Verification items for the finished model (mm, model axes). Face numbers are marked on the shaded views. A direction names the side the tool comes from. Coordinates: 2 decimals unless noted, no trailing zeros. Write each loop counter-clockwise with the first axis right and the second up, starting at its lowest first coordinate (ties: lowest second). Pieces come first, ordered by that corner, then holes. Notation, with made-up numbers: (78, 15.25) -> (85, 15.25) arc R22 ccw to (85, 28.25) -> close; hole circle Ø5 at (25.25, 26). An arc over 180 degrees is marked (long way). Answer in a Markdown table with one row per item.
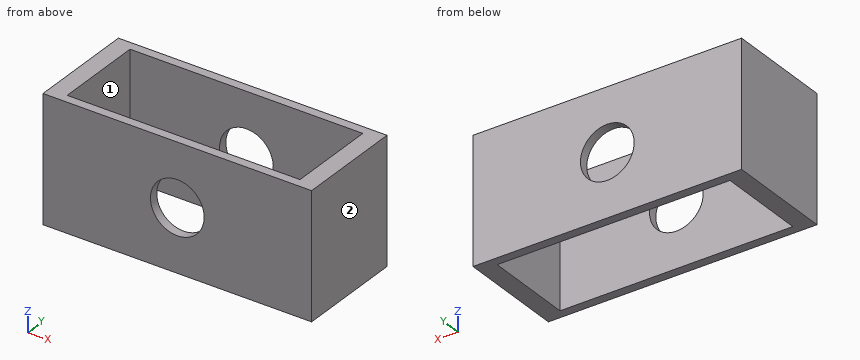
```python
from build123d import *

# Parameters (mm, degrees)
SKETCH_1_W      = 30
SKETCH_1_H      = 14
SKETCH_1_R      = 3
EXTRUDE_1_DEPTH = 1
SKETCH_2_W      = 2
SKETCH_2_H      = 14
EXTRUDE_2_DEPTH = 10
SKETCH_3_W      = 30
SKETCH_3_H      = 14
SKETCH_3_R      = 3
EXTRUDE_3_DEPTH = 1


with BuildPart() as part:
    # Эскиз1 → Бобышка-Вытянуть1 (new body)
    with BuildSketch(Plane(origin=(0, 0, 0), x_dir=(1, 0, 0), z_dir=(0, 1, 0))):
        Rectangle(SKETCH_1_W, SKETCH_1_H)
        with Locations(Location((0, 0, 0), (0, 0, 270))):
            Circle(SKETCH_1_R, mode=Mode.SUBTRACT)
    extrude(amount=EXTRUDE_1_DEPTH)

    # Эскиз2 → Бобышка-Вытянуть2 (add)
    with BuildSketch(Plane(origin=(0, 1, 0), x_dir=(1, 0, 0), z_dir=(0, 1, 0))):
        with Locations((-14, 0)):
            Rectangle(SKETCH_2_W, SKETCH_2_H)
        with Locations((14, 0)):
            Rectangle(SKETCH_2_W, SKETCH_2_H)
    extrude(amount=EXTRUDE_2_DEPTH)

    # Эскиз3 → Бобышка-Вытянуть3 (add)
    with BuildSketch(Plane(origin=(0, 11, 0), x_dir=(1, 0, 0), z_dir=(0, 1, 0))):
        Rectangle(SKETCH_3_W, SKETCH_3_H)
        with Locations(Location((0, 0, 0), (0, 0, 270))):
            Circle(SKETCH_3_R, mode=Mode.SUBTRACT)
    extrude(amount=EXTRUDE_3_DEPTH)


solid = part.part
```
1. Depth check by flat-ended pin: P1, Ø4, axis at x = 3.5, z = -4.5, coming from the -Y side; P2, Ø3.5, axis at x = 0, z = 0, coming from the -Y side. Enter the tip coordinate at first touch or a pass-through.
Geometry says:
| item | result |
|---|---|
| P1 | y = 0 |
| P2 | through |
2. Section check B-B, the plane y = 3. Record the boundary of the cut face in (x, z), plus the area to 3 significant figures.
Geometry says:
| item | result |
|---|---|
| outline | (-15, -7) -> (-13, -7) -> (-13, 7) -> (-15, 7) -> close; (13, -7) -> (15, -7) -> (15, 7) -> (13, 7) -> close |
| area | 56.0 mm^2 |
3. Section check C-C, the plane z = 0. Record the boundary of the cut face in (x, y), plus the area to 3 significant figures.
Geometry says:
| item | result |
|---|---|
| outline | (-15, 0) -> (-3, 0) -> (-3, 1) -> (-13, 1) -> (-13, 11) -> (-3, 11) -> (-3, 12) -> (-15, 12) -> close; (3, 0) -> (15, 0) -> (15, 12) -> (3, 12) -> (3, 11) -> (13, 11) -> (13, 1) -> (3, 1) -> close |
| area | 88.0 mm^2 |
4. Tool access check on the marked faces 1 and 2. Record the directions out of +Z, -Z, +X, -X, +Y, -Y that give a thin tool (end or side, any length) a straight path to the whole face; none if there is none.
Geometry says:
| item | result |
|---|---|
| face 1 | +Z, -Z |
| face 2 | +Z, -Z, +X, +Y, -Y |
5. Section check A-A, the plane x = 0. Record the boundary of the cut face in (y, z).
Geometry says:
| item | result |
|---|---|
| outline | (0, -7) -> (1, -7) -> (1, -3) -> (0, -3) -> close; (0, 3) -> (1, 3) -> (1, 7) -> (0, 7) -> close; (11, -7) -> (12, -7) -> (12, -3) -> (11, -3) -> close; (11, 3) -> (12, 3) -> (12, 7) -> (11, 7) -> close |
6. Section check D-D, the plane x = -8.25. Record the boundary of the cut face in (y, z).
Geometry says:
| item | result |
|---|---|
| outline | (0, -7) -> (1, -7) -> (1, 7) -> (0, 7) -> close; (11, -7) -> (12, -7) -> (12, 7) -> (11, 7) -> close |
7. Thickness scan on line 1 (X direction, y = 2.5, z = -2.5); line 2 (Y direction, x = -4.25, z = -4.75); line 3 (X direction, y = 11.75, z = 0). Record the ranges inside material, lowest first. Write a range as from..to.
Geometry says:
| item | result |
|---|---|
| line 1 | -15..-13, 13..15 |
| line 2 | 0..1, 11..12 |
| line 3 | -15..-3, 3..15 |
